Autodesk Inventor part; units mm, degrees
ref_plane "YZ Plane" through (0, 0, 0) normal (1, 0, 0) x (0, 1, 0)
ref_plane "XZ Plane" through (0, 0, 0) normal (0, 1, 0) x (-1, 0, 0)
ref_plane "XY Plane" through (0, 0, 0) normal (0, 0, 1) x (1, 0, 0)
sketch "Sketch1" plane through (0, 0, 0) normal (0, 0, 1) x (1, 0, 0)
  arc A0 (-114.2223, -38.8548) -> (0, -120.65) centre (0, 0) ccw
  line L0 (-120.65, 0) -> (-121.2596, 0)
  line L1 (120.65, 0) -> (121.2596, 0)
  line L2 (-121.2596, 0) -> (-121.2596, -25.4)
  line L3 (-120.65, 0) -> (-120.65, -25.4)
  line L4 (-121.2596, -25.4) -> (-120.65, -30.3117) construction
  line L5 (-120.65, -30.3117) -> (-117.4666, -33.4581) construction
  line L6 (-117.4666, -33.4581) -> (-114.5061, -39.9028) construction
  spline S0 degree 3 poles (-121.2596, -25.4) (-120.65, -30.3117) (-117.4666, -33.4581) (-114.5061, -39.9028) knots 1 1 1 1 2 2 2 2
  line L7 (-120.65, -25.4) -> (-120.1784, -29.1998) construction
  line L8 (-120.1784, -29.1998) -> (-116.9951, -32.3462) construction
  line L9 (-116.9951, -32.3462) -> (-114.2223, -38.8548) construction
  spline S1 degree 3 poles (-120.65, -25.4) (-120.1784, -29.1998) (-116.9951, -32.3462) (-114.2223, -38.8548) knots 1 1 1 1 2 2 2 2
  arc A1 (-114.5061, -39.9028) -> (0, -121.2596) centre (0, 0) ccw
  line L10 (0, 0) -> (0, -121.2596)
  arc A2 (0, -120.65) -> (114.2223, -38.8548) centre (0, 0) ccw
  line L11 (120.65, 0) -> (121.2596, 0)
  line L12 (121.2596, 0) -> (121.2596, -25.4)
  line L13 (120.65, 0) -> (120.65, -25.4)
  line L14 (121.2596, -25.4) -> (120.65, -30.3117) construction
  line L15 (120.65, -30.3117) -> (117.4666, -33.4581) construction
  line L16 (117.4666, -33.4581) -> (114.5061, -39.9028) construction
  spline S2 degree 3 poles (121.2596, -25.4) (120.65, -30.3117) (117.4666, -33.4581) (114.5061, -39.9028) knots 1 1 1 1 2 2 2 2
  spline S3 degree 3 poles (120.65, -25.4) (120.1784, -29.1998) (116.9951, -32.3462) (114.2223, -38.8548) knots 1 1 1 1 2 2 2 2
  line L17 (120.65, -25.4) -> (120.1784, -29.1998) construction
  line L18 (120.1784, -29.1998) -> (116.9951, -32.3462) construction
  line L19 (116.9951, -32.3462) -> (114.2223, -38.8548) construction
  arc A3 (0, -121.2596) -> (114.5061, -39.9028) centre (0, 0) ccw
  dimension "d0" = 241.3
  dimension "d1" = 0.6096
  dimension "d2" = 0.6096
  dimension "d5" = 25.4
  dimension "d6" = 25.4
  dimension "d7" = 1.1119
  dimension "d8" = 1.1119
  dimension "d9" = 3.1463
  dimension "d10" = 3.1833
  dimension "d11" = 0.6096
  dimension "d12" = 3.1833
  dimension "d14" = 14.5028
  dimension "d15" = 3.7998
extrude "Extrusion1" add sketch "Sketch1" against normal blind 508
sketch "Sketch2" plane through (-120.65, -25.4, 0) normal (1, 0, 0) x (0, 0, -1)
  line L0 (0, 25.4) -> (0, 0)
  line L1 (0, 25.4) -> (508, 25.4)
  line L2 (508, 0) -> (508, 25.4)
  line L3 (0, 0) -> (508, 0)
  circle A0 centre (12.7, 12.7) radius 2.413
  circle A1 centre (254, 12.7) radius 2.413
  circle A2 centre (495.3, 12.7) radius 2.413
  dimension "d18" = 4.826
  dimension "d19" = 12.7
  dimension "d20" = 12.7
  dimension "d23" = 241.3
extrude "Extrusion2" cut sketch "Sketch2" along normal mid plane 560.3875 contours A0 | A1 | A2
properties part number "Ballslide"
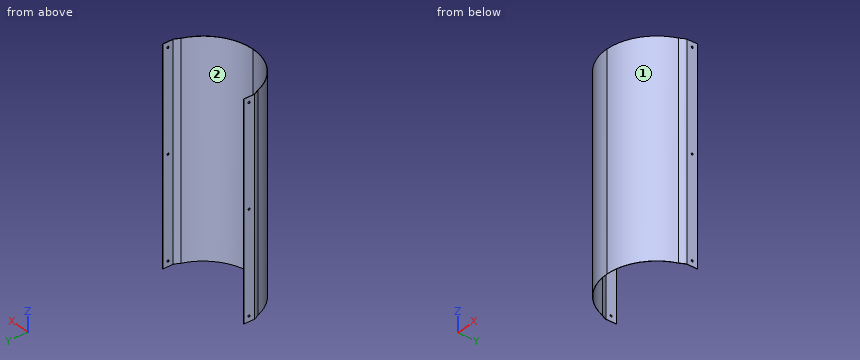
Verification items for the finished model (mm, model axes). Face numbers are marked on the shaded views. Coordinates: 2 decimals unless noted, no trailing zeros. Order: outer loops, then holes, each group sorted by start corner. A loop starts at its lowest first (then second) coordinate and runs counter-clockwise, first axis right, second up.
1. Sectioned sample at C-C, the plane x = 80.5. Record the cut outline in (y, z), and give its area (3 significant figures).
Results found:
outline: (-90.68, -508) - (-89.87, -508) - (-89.87, 0) - (-90.68, 0) - close
area: 415 mm2
2. Sectioned sample at B-B, the plane y = -75. Record the cut outline in (x, z).
Results found:
outline: (-95.28, -508) - (-94.51, -508) - (-94.51, 0) - (-95.28, 0) - close; (94.51, -508) - (95.28, -508) - (95.28, 0) - (94.51, 0) - close
3. Release check for a two-part mould opening along X. For the marked faces 1 and 2 record: +X half, -X half, draft (parallel to the pull), parting line (faces both ways), or undercut.
Results found:
face 1: +X half
face 2: undercut
4. Scan lines: line 1 (X direction, y = -25, z = -454); line 2 (X direction, y = -108, z = -229); line 3 (Y direction, x = -53.5, z = -201). Record each from-to range of solid material in increasing order.
Results found:
line 1: x = -121.26 to -120.65, 120.65 to 121.26
line 2: x = -55.14 to -53.78, 53.78 to 55.14
line 3: y = -108.82 to -108.14
5. Go/stop test with flat-tipped pins: pin 1 Ø1 at (y, z) = (-82, -448.5) entering from -X; pin 2 Ø1 at (x, z) = (6.5, -447.5) entering from +Y; pin 3 Ø3 at (y, z) = (-64, -313) entering from -X. Record where each tip stops, or that it passes through.
Results found:
pin 1: stops at x = -89.79
pin 2: stops at y = -120.45
pin 3: stops at x = -103.91
6. Sectioned sample at A-A, the plane y = -101.5. Record the cut outline in (x, z), and give its area (3 significant figures).
Results found:
outline: (-66.34, -508) - (-65.22, -508) - (-65.22, 0) - (-66.34, 0) - close; (65.22, -508) - (66.34, -508) - (66.34, 0) - (65.22, 0) - close
area: 1,140 mm2
7. Sectioned sample at D-D, the plane x = -65. Record the cut outline in (y, z), and give its area (3 significant figures).
Results found:
outline: (-102.37, -508) - (-101.64, -508) - (-101.64, 0) - (-102.37, 0) - close
area: 367 mm2
